Part model, mm, in its own coordinate system. Face numbers are marked on the shaded views. A direction names the side the tool comes from. Give positions to 0.01 mm unless a question says otherwise; leave off trailing zeros. Order: outer loops, then holes, each group sorted by start corner. A loop starts at its lowest first (then second) coordinate and runs counter-clockwise, first axis right, second up. Notation, with made-up numbers: (-11, 10.5) - (-2, 10.5) arc R11 cw to (-2, 20.5) - close; hole circle Ø10 at (-19.75, 58). An arc over 180 degrees is marked (long way). Use one line per item in the form item = value. Start each with the question number.
1. Drill centre lines: line 1 (Y direction, x = -5, z = 2.7); line 2 (Y direction, x = -19, z = 1.3); line 3 (X direction, y = -14.5, z = 2.6). Where is each one in solid material? Low to high.
2. Pull direction Y, two halves, no side cores. Call the marked faces 1, 2 and 3: +Y half, -Y half, draft (parallel to the pull), parting line (faces both ways), or undercut.
3. Tool access for the marked faces 4, 5, 6, 7 and 8: list every direction of +Z, -Z, +X, -X, +Y, -Y with a clear straight run to the whole face (end or side of a thin tool).
4. Pin check, flat tips, straight feed: P1, Ø1.5, axis at y = 7, z = 1.5, coming from the +X side; P2, Ø1.5, axis at x = -23.5, z = 2, coming from the -Y side; P3, Ø2.5, axis at x = -7.28, y = -24, coming from the +Z side (1 decimal); P4, Ø0.9, axis at x = -26, z = 1, coming from the +Y side. Stop position of each tip, or through.
5. Band-saw the part on B-B, the plane y = -13.5. List the corners of the cut face in (x, z), plus the area to 3 significant figures.
6. Band-saw the part on A-A, the plane z = 2.25. State how many separate pieces and enclosed holes the cut face has, plus the area to 3 significant figures.
7. Band-saw the part on D-D, the plane x = 1.5. List the corners of the cut face in (y, z), plus the area to 3 significant figures.
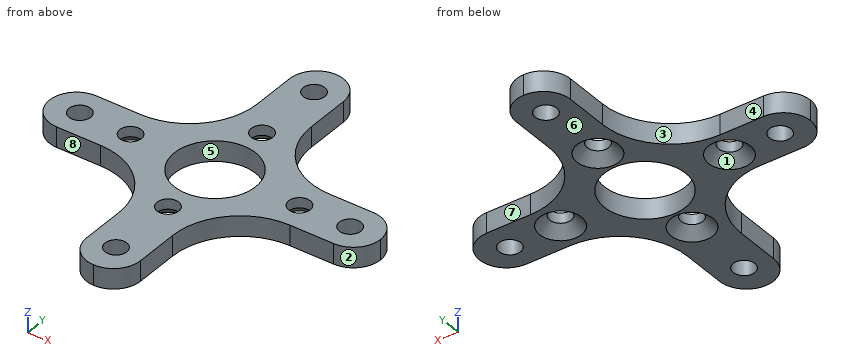
from build123d import *

# Parameters (mm, degrees)
BOSS_EXTRU_1_DEPTH      = 3
ENL_V_MAT_EXTRU_1_REACH = 44.796
ESQUISSE2_R             = 1.6
CONG_1_R                = 10
CONG_2_R                = 4
ENL_V_MAT_EXTRU_2_REACH = 44.796
ESQUISSE3_R             = 6
CHANFREIN1_SIZE         = 1.5


with BuildPart() as part:
    # Esquisse1 → Boss.-Extru.1 (new body)
    with BuildSketch(Plane.XY):
        Polygon((-11.28415855, 20.5), (-11.28415855, 0), (-31.78415855, 0), (-31.78415855, -8), (-11.28415855, -8), (-11.28415855, -28.5), (-3.28415855, -28.5), (-3.28415855, -8), (17.21584145, -8), (17.21584145, 0), (-3.28415855, 0), (-3.28415855, 20.5), align=None)
    extrude(amount=BOSS_EXTRU_1_DEPTH)

    # Esquisse2 → Enlèv. mat.-Extru.1 (cut, up to next)
    with BuildSketch(Plane.XY.offset(3), mode=Mode.PRIVATE) as enl_v_mat_extru_1_sk1:
        with Locations((-27.28415855, -4)):
            Circle(ESQUISSE2_R)
    enl_v_mat_extru_1_tool1 = extrude(enl_v_mat_extru_1_sk1.sketch, amount=-ENL_V_MAT_EXTRU_1_REACH, mode=Mode.PRIVATE) & part.part
    # Esquisse2 → Enlèv. mat.-Extru.1 (cut, up to next)
    with BuildSketch(Plane.XY.offset(3), mode=Mode.PRIVATE) as enl_v_mat_extru_1_sk2:
        with Locations((-19.78415855, -4)):
            Circle(ESQUISSE2_R)
    enl_v_mat_extru_1_tool2 = extrude(enl_v_mat_extru_1_sk2.sketch, amount=-ENL_V_MAT_EXTRU_1_REACH, mode=Mode.PRIVATE) & part.part
    # Esquisse2 → Enlèv. mat.-Extru.1 (cut, up to next)
    with BuildSketch(Plane.XY.offset(3), mode=Mode.PRIVATE) as enl_v_mat_extru_1_sk3:
        with Locations((-7.28415855, -13.5)):
            Circle(ESQUISSE2_R)
    enl_v_mat_extru_1_tool3 = extrude(enl_v_mat_extru_1_sk3.sketch, amount=-ENL_V_MAT_EXTRU_1_REACH, mode=Mode.PRIVATE) & part.part
    # Esquisse2 → Enlèv. mat.-Extru.1 (cut, up to next)
    with BuildSketch(Plane.XY.offset(3), mode=Mode.PRIVATE) as enl_v_mat_extru_1_sk4:
        with Locations((-7.28415855, 5.5)):
            Circle(ESQUISSE2_R)
    enl_v_mat_extru_1_tool4 = extrude(enl_v_mat_extru_1_sk4.sketch, amount=-ENL_V_MAT_EXTRU_1_REACH, mode=Mode.PRIVATE) & part.part
    # Esquisse2 → Enlèv. mat.-Extru.1 (cut, up to next)
    with BuildSketch(Plane.XY.offset(3), mode=Mode.PRIVATE) as enl_v_mat_extru_1_sk5:
        with Locations((-7.28415855, 16)):
            Circle(ESQUISSE2_R)
    enl_v_mat_extru_1_tool5 = extrude(enl_v_mat_extru_1_sk5.sketch, amount=-ENL_V_MAT_EXTRU_1_REACH, mode=Mode.PRIVATE) & part.part
    # Esquisse2 → Enlèv. mat.-Extru.1 (cut, up to next)
    with BuildSketch(Plane.XY.offset(3), mode=Mode.PRIVATE) as enl_v_mat_extru_1_sk6:
        with Locations((5.21584145, -4)):
            Circle(ESQUISSE2_R)
    enl_v_mat_extru_1_tool6 = extrude(enl_v_mat_extru_1_sk6.sketch, amount=-ENL_V_MAT_EXTRU_1_REACH, mode=Mode.PRIVATE) & part.part
    # Esquisse2 → Enlèv. mat.-Extru.1 (cut, up to next)
    with BuildSketch(Plane.XY.offset(3), mode=Mode.PRIVATE) as enl_v_mat_extru_1_sk7:
        with Locations((12.71584145, -4)):
            Circle(ESQUISSE2_R)
    enl_v_mat_extru_1_tool7 = extrude(enl_v_mat_extru_1_sk7.sketch, amount=-ENL_V_MAT_EXTRU_1_REACH, mode=Mode.PRIVATE) & part.part
    # Esquisse2 → Enlèv. mat.-Extru.1 (cut, up to next)
    with BuildSketch(Plane.XY.offset(3), mode=Mode.PRIVATE) as enl_v_mat_extru_1_sk8:
        with Locations((-7.28415855, -24)):
            Circle(ESQUISSE2_R)
    enl_v_mat_extru_1_tool8 = extrude(enl_v_mat_extru_1_sk8.sketch, amount=-ENL_V_MAT_EXTRU_1_REACH, mode=Mode.PRIVATE) & part.part
    add(enl_v_mat_extru_1_tool1.solids().sort_by_distance((-27.284159, -4, 3))[0], mode=Mode.SUBTRACT)
    add(enl_v_mat_extru_1_tool2.solids().sort_by_distance((-19.784159, -4, 3))[0], mode=Mode.SUBTRACT)
    add(enl_v_mat_extru_1_tool3.solids().sort_by_distance((-7.284159, -13.5, 3))[0], mode=Mode.SUBTRACT)
    add(enl_v_mat_extru_1_tool4.solids().sort_by_distance((-7.284159, 5.5, 3))[0], mode=Mode.SUBTRACT)
    add(enl_v_mat_extru_1_tool5.solids().sort_by_distance((-7.284159, 16, 3))[0], mode=Mode.SUBTRACT)
    add(enl_v_mat_extru_1_tool6.solids().sort_by_distance((5.215841, -4, 3))[0], mode=Mode.SUBTRACT)
    add(enl_v_mat_extru_1_tool7.solids().sort_by_distance((12.715841, -4, 3))[0], mode=Mode.SUBTRACT)
    add(enl_v_mat_extru_1_tool8.solids().sort_by_distance((-7.284159, -24, 3))[0], mode=Mode.SUBTRACT)

    # Congé1
    cong_1_edges = [part.edges().sort_by_distance(p)[0] for p in [
        (-3.28415855, 0, 1.5),
        (-3.28415855, -8, 1.5),
        (-11.28415855, -8, 1.5),
        (-11.28415855, 0, 1.5),
    ]]
    fillet(cong_1_edges, radius=CONG_1_R)

    # Congé2
    cong_2_edges = [part.edges().sort_by_distance(p)[0] for p in [
        (-11.28415855, -28.5, 1.5),
        (-3.28415855, -28.5, 1.5),
        (17.21584145, -8, 1.5),
        (17.21584145, 0, 1.5),
        (-3.28415855, 20.5, 1.5),
        (-11.28415855, 20.5, 1.5),
        (-31.78415855, -8, 1.5),
        (-31.78415855, 0, 1.5),
    ]]
    fillet(cong_2_edges, radius=CONG_2_R - 0.0001)  # a hair under: the kernel refuses the full size

    # Esquisse3 → Enlèv. mat.-Extru.2 (cut, up to next)
    with BuildSketch(Plane(origin=(0, 0, 0), x_dir=(-1, 0, 0), z_dir=(0, 0, -1)), mode=Mode.PRIVATE) as enl_v_mat_extru_2_sk1:
        with Locations((7.28415855, -4)):
            Circle(ESQUISSE3_R)
    enl_v_mat_extru_2_tool1 = extrude(enl_v_mat_extru_2_sk1.sketch, amount=-ENL_V_MAT_EXTRU_2_REACH, mode=Mode.PRIVATE) & part.part
    add(enl_v_mat_extru_2_tool1.solids().sort_by_distance((-7.284159, -4, 0))[0], mode=Mode.SUBTRACT)

    # Chanfrein1
    chanfrein1_edges = [part.edges().sort_by_distance(p)[0] for p in [
        (3.61584145, -4, 0),
        (-8.88415855, 5.5, 0),
        (-8.88415855, -13.5, 0),
        (-21.38415855, -4, 0),
    ]]
    chamfer(chanfrein1_edges, length=CHANFREIN1_SIZE)


solid = part.part
From the geometry:
q1.line_1 = -27.78 to -9.55, 1.55 to 19.78
q1.line_2 = -8.26 to -5.62, -2.38 to 0.26
q1.line_3 = -11.92 to -8.53, -6.04 to -2.65
q2.face_1 = undercut
q2.face_2 = -Y half
q2.face_3 = +Y half
q3.face_4 = +Z, -Z, -X, +Y
q3.face_5 = +Z, -Z
q3.face_6 = -Z, +X, -X, +Y, -Y
q3.face_7 = +Z, -Z, +X, +Y
q3.face_8 = +Z, -Z, -X, -Y
q4.P1 = -2.55
q4.P2 = -8
q4.P3 = through
q4.P4 = 0
q5.outline = (-12.35, 0) - (-10.38, 0) - (-8.88, 1.5) - (-8.88, 3) - (-12.35, 3) - close; (-5.68, 1.5) - (-4.18, 0) - (-2.21, 0) - (-2.21, 3) - (-5.68, 3) - close
q5.area = 18.6 mm²
q6.separate_pieces = 1
q6.enclosed_holes = 9
q6.area = 601 mm²
q7.outline = (-9.47, 0) - (1.47, 0) - (1.47, 3) - (-9.47, 3) - close
q7.area = 32.8 mm²
